Print and shaded views of the part. All mm, measured from the part's lowest x, y and z. Round coordinates to 2 decimals unless told otherwise and drop trailing zeros. Loops run counter-clockwise (first coordinate to the right, second up) from the corner with the lowest first, then second, coordinate; pieces in that order, holes last. Notation, with made-up numbers: (31.5, 13.5) - (71.5, 13.5) arc R10 ccw to (71.5, 32.5) - close; hole circle Ø9 at (9, -30). An arc over 180 degrees is marked (long way). Use one line per item in the form item = value.
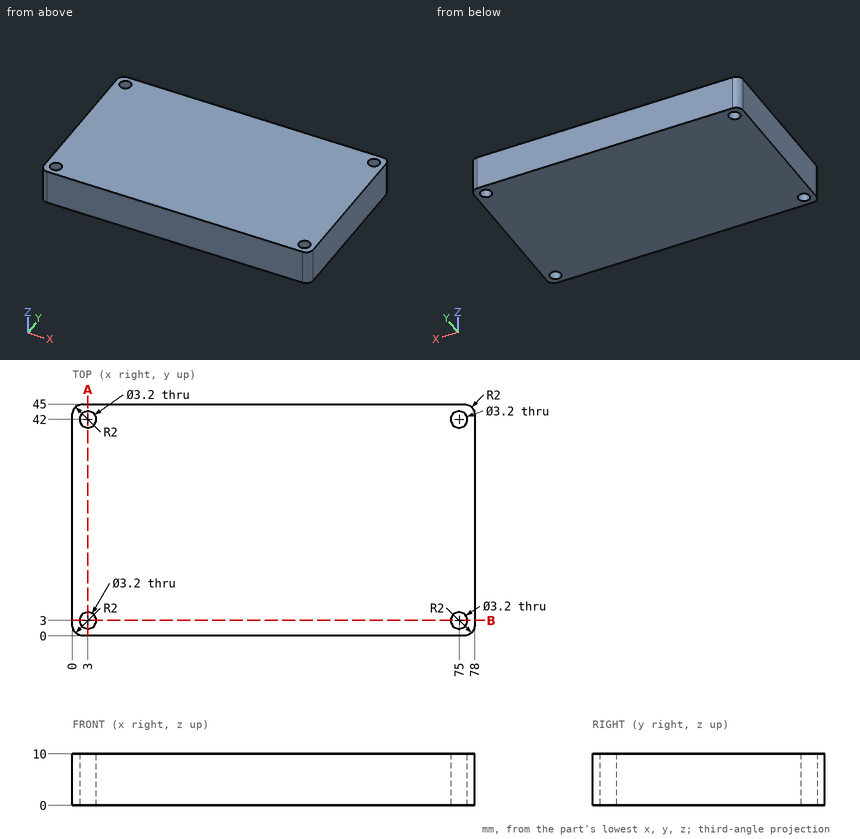
1. Cut at A-A, the plane x = 3. Give the cut face in (y, z).
Geometry check:
outline = (0, 0) - (1.4, 0) - (1.4, 10) - (0, 10) - close; (4.6, 0) - (40.4, 0) - (40.4, 10) - (4.6, 10) - close; (43.6, 0) - (45, 0) - (45, 10) - (43.6, 10) - close
2. Flat gauge pin, fed straight in: pin 1 (1.9 mm diameter, centred on x = 75, y = 42, fed in from +Z). Where does the tip first touch, or does it go through?
Geometry check:
pin_1 = through
3. Cut at B-B, the plane y = 3. Give the cut face in (x, z), plus the area to 3 significant figures.
Geometry check:
outline = (0, 0) - (1.4, 0) - (1.4, 10) - (0, 10) - close; (4.6, 0) - (73.4, 0) - (73.4, 10) - (4.6, 10) - close; (76.6, 0) - (78, 0) - (78, 10) - (76.6, 10) - close
area = 716 mm^2
4. Wall check: probe 1 along Y at (x, z) = (75, 7.5). Give the ranges that are in metal, low to high.
Geometry check:
probe_1 = 0 to 1.4, 4.6 to 40.4, 43.6 to 45
